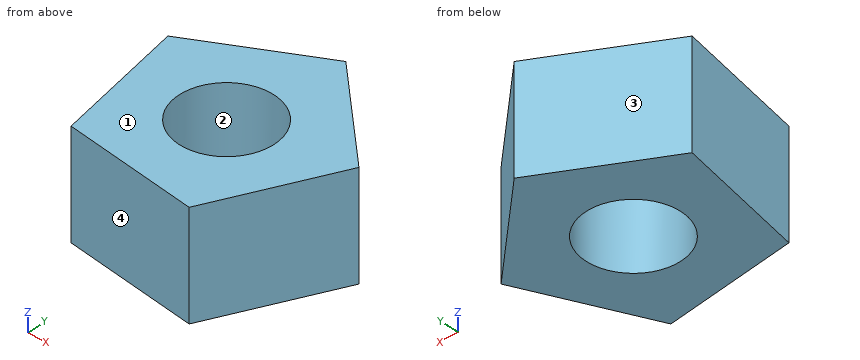
from build123d import *

# Parameters (mm, degrees)
F0_R     = 56.77758
F1_DEPTH = 127


with BuildPart() as f1:
    # F0 (on Top) → F1 (new body)
    with BuildSketch(Plane.XY):
        Polygon((16.924353, 137.300746), (-125.350856, 58.52428), (-94.395442, -101.130752), (67.011265, -121.026522), (135.810682, 26.332248), align=None)
        Circle(F0_R, mode=Mode.SUBTRACT)
    extrude(amount=F1_DEPTH)


solid = f1.part
Can you work these out from the model? Positions are in its coordinate system, mm. Face numbers are marked on the shaded views. Give positions to 0.01 mm unless a question says otherwise; leave off trailing zeros. Write each loop counter-clockwise with the first axis right and the second up, starting at its lowest first coordinate (ties: lowest second). Pieces come first, ordered by that corner, then holes. Notation, with made-up numbers: (36, -4.5) -> (77, -4.5) arc R30 ccw to (77, 28.5) -> close; hole circle Ø5 at (46.25, 61). An arc over 180 degrees is marked (long way). Answer as a JSON object with one key per item and string values. Group by question number.
Item 1: Please list where these lines run through material, in increasing order: line 1 (Y direction, x = 0, z = 36); line 2 (Y direction, x = 50, z = 8); line 3 (X direction, y = 27, z = 55). Write a range as [from, to].
Item 2: Suppose I cut it at D-D (y = 88). Please give me the cut outline in (x, z), plus the area to 3 significant figures.
Item 3: I'm going to push flat-ended pins straight in: P1, Ø10, axis at y = 87.5, z = 94.5, coming from the -X side; P2, Ø3, axis at x = 90.5, z = 13, coming from the -Y side; P3, Ø1, axis at x = -49, z = 18.5, coming from the +Y side. Where does each tip first touch, or does it pass through?
Item 4: Suppose I cut it at B-B (z = 50.5). Please give me the cut outline in (x, y), plus the area to 3 significant figures.
Item 5: We'd pull the mould along Y, two halves only. Please class the marked faces 1, 2, 3 and 4: +Y half, -Y half, draft (parallel to the pull), parting line (faces both ways), or undercut.
Item 6: Suppose I cut it at A-A (x = -37). Please give me the cut outline in (y, z), plus the area to 3 significant figures.
Item 7: Suppose I cut it at C-C (y = -45). Please give me the cut outline in (x, z).
Findings:
{
 "1": {"line 1": "y = [-112.77, -56.78], [56.78, 127.93]", "line 2": "y = [-118.93, -26.9], [26.9, 106.43]", "line 3": "x = [-119.24, -49.95], [49.95, 135.1]"},
 "2": {"outline": "(-72.12, 0) -> (69.74, 0) -> (69.74, 127) -> (-72.12, 127) -> close", "area": "18,000 mm²"},
 "3": {"P1": "stops at x = -82.05", "P2": "stops at y = -73.93", "P3": "stops at y = 101.08"},
 "4": {"outline": "(-125.35, 58.52) -> (-94.4, -101.13) -> (67.01, -121.03) -> (135.81, 26.33) -> (16.92, 137.3) -> close; hole circle Ø113.56 at (0, 0)", "area": "35,400 mm²"},
 "5": {"face 1": "draft", "face 2": "undercut", "face 3": "+Y half", "face 4": "-Y half"},
 "6": {"outline": "(-108.21, 0) -> (-43.07, 0) -> (-43.07, 127) -> (-108.21, 127) -> close; (43.07, 0) -> (107.44, 0) -> (107.44, 127) -> (43.07, 127) -> close", "area": "16,400 mm²"},
 "7": {"outline": "(-105.28, 0) -> (-34.62, 0) -> (-34.62, 127) -> (-105.28, 127) -> close; (34.62, 0) -> (102.51, 0) -> (102.51, 127) -> (34.62, 127) -> close"}
}
